Design review of the part shown in the three views and the two pictorial views. Dimensions are in mm from the part's minimum x, y and z. Give positions to 0.01 mm unless a question says otherwise; leave off trailing zeros. Loops run counter-clockwise (first coordinate to the right, second up) from the corner with the lowest first, then second, coordinate; pieces in that order, holes last.
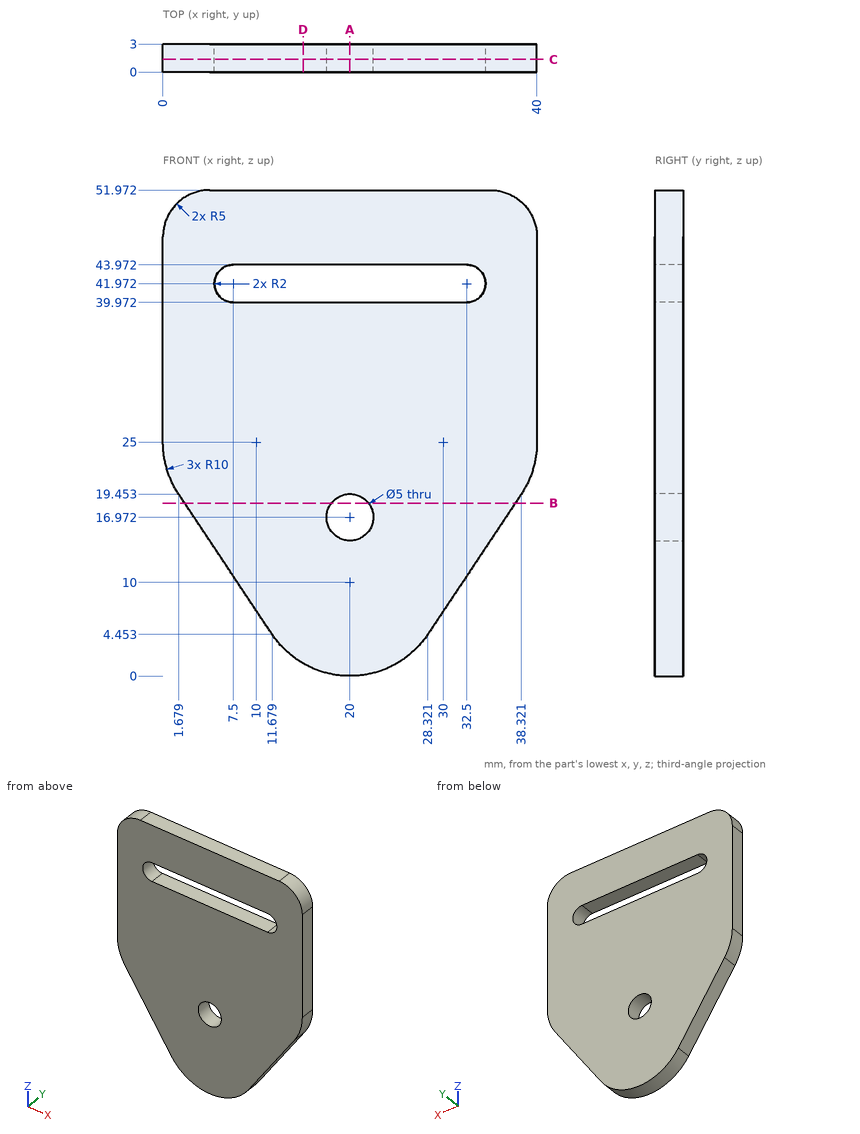
Q1. Consider section C-C on y = 1.35. Give the boundary of the cut face in (x, z), plus the area to 3 significant figures.
Answers:
outline: (0, 25) arc R10 ccw to (1.68, 19.45) - (11.68, 4.45) arc R10 ccw to (28.32, 4.45) - (38.32, 19.45) arc R10 ccw to (40, 25) - (40, 46.97) arc R5 ccw to (35, 51.97) - (5, 51.97) arc R5 ccw to (0, 46.97) - close; hole (7.5, 39.97) - (32.5, 39.97) arc R2 ccw to (32.5, 43.97) - (7.5, 43.97) arc R2 ccw to start; hole circle Ø5 at (20, 16.97)
area: 1,600 mm2
Q2. For probe 1 along Z at (x, y) = (10.5, 2.3) (1 decimal); probe 2 along X at (y, z) = (1.8, 43) (1 decimal); probe 3 along Z at (x, y) = (27, 2.5) (1 decimal), list the stretches that pass through material, from the lowest coordinate up.
Answers:
probe 1: z = 6.2 to 40, 44 to 52
probe 2: x = 0 to 5.8, 34.2 to 40
probe 3: z = 2.9 to 40, 44 to 52
Q3. Consider section A-A on x = 20. Give the boundary of the cut face in (y, z).
Answers:
outline: (0, 0) - (3, 0) - (3, 14.47) - (0, 14.47) - close; (0, 19.47) - (3, 19.47) - (3, 39.97) - (0, 39.97) - close; (0, 43.97) - (3, 43.97) - (3, 51.97) - (0, 51.97) - close
Q4. Consider section B-B on z = 18.5. Give the boundary of the cut face in (x, y) (1 decimal).
Answers:
outline: (2.3, 0) - (18, 0) - (18, 3) - (2.3, 3) - close; (22, 0) - (37.7, 0) - (37.7, 3) - (22, 3) - close
Q5. Consider section D-D on x = 15. Give the boundary of the cut face in (y, z), plus the area to 3 significant figures.
Answers:
outline: (0, 1.34) - (3, 1.34) - (3, 39.97) - (0, 39.97) - close; (0, 43.97) - (3, 43.97) - (3, 51.97) - (0, 51.97) - close
area: 140 mm2
Q6. For pin 1 Ø4 at (x, z) = (20, 16.97) entering from +Y; pin 2 Ø1 at (x, y) = (21, 0.5) entering from -Z, all flat-tipped, find the tip position at first contact; note any pin that passes through.
Answers:
pin 1: passes through
pin 2: stops at z = 0.01
